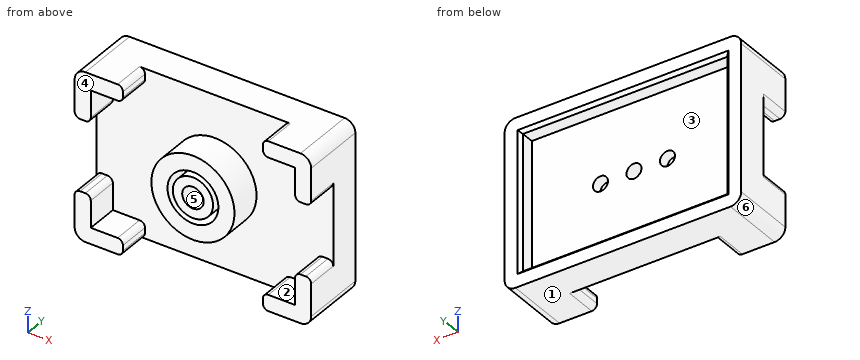
```python
from build123d import *

# Parameters (mm, degrees)
F0_R     = 9.5
F0_R_2   = 7.75
F0_R_3   = 1.4
F0_R_4   = 4.75
F0_R_5   = 3.75
F0_R_6   = 2
F1_DEPTH = 3
F0_W     = 26.1
F0_H     = 3
F0_W_2   = 3
F0_H_2   = 13.3
F2_DEPTH = 6
F3_DEPTH = 1
F4_DEPTH = 6
F5_DEPTH = 6
F6_DEPTH = 6
F7_SIZE  = 0.6
F8_DEPTH = 3
F9_R     = 2
F10_SIZE = 0.4
F11_R    = 1


with BuildPart() as f1:
    # F0 (on Front) → F1 (new body)
    with BuildSketch(Plane.XZ):
        Polygon((-13.05, 12.65), (-19.05, 12.65), (-19.05, 6.65), (-19.05, -6.65), (-19.05, -12.65), (-13.05, -12.65), (13.05, -12.65), (19.05, -12.65), (19.05, -6.65), (19.05, 6.65), (19.05, 12.65), (13.05, 12.65), align=None)
        Circle(F0_R, mode=Mode.SUBTRACT)
        Circle(F0_R)
        Circle(F0_R_2, mode=Mode.SUBTRACT)
        Circle(F0_R_2)
        with Locations((-6.25, 0)):
            Circle(F0_R_3, mode=Mode.SUBTRACT)
        Circle(F0_R_4, mode=Mode.SUBTRACT)
        with Locations((6.25, 0)):
            Circle(F0_R_3, mode=Mode.SUBTRACT)
        Circle(F0_R_4)
        Circle(F0_R_5, mode=Mode.SUBTRACT)
        Circle(F0_R_5)
        Circle(F0_R_6, mode=Mode.SUBTRACT)
    extrude(amount=-F1_DEPTH)

    # F0 (on Front) → F2 (join)
    with BuildSketch(Plane.XZ):
        Polygon((-19.05, 6.65), (-19.05, 12.65), (-13.05, 12.65), (-13.05, 15.65), (-22.05, 15.65), (-22.05, 6.65), align=None)
        Polygon((13.05, 15.65), (13.05, 12.65), (19.05, 12.65), (19.05, 6.65), (22.05, 6.65), (22.05, 15.65), align=None)
        with Locations((0, -14.15)):
            Rectangle(F0_W, F0_H)
        with Locations((0, 14.15)):
            Rectangle(F0_W, F0_H)
        with Locations((-20.55, 0)):
            Rectangle(F0_W_2, F0_H_2)
        Polygon((-19.05, -12.65), (-19.05, -6.65), (-22.05, -6.65), (-22.05, -15.65), (-13.05, -15.65), (-13.05, -12.65), align=None)
        Polygon((22.05, -6.65), (19.05, -6.65), (19.05, -12.65), (13.05, -12.65), (13.05, -15.65), (22.05, -15.65), align=None)
        with Locations((20.55, 0)):
            Rectangle(F0_W_2, F0_H_2)
    extrude(amount=-F2_DEPTH)

    # F0 (on Front) → F3 (join)
    with BuildSketch(Plane.XZ):
        with Locations((-6.25, 0)):
            Circle(F0_R_3)
        with Locations((6.25, 0)):
            Circle(F0_R_3)
    extrude(amount=-F3_DEPTH)

    # F0 (on Front) → F4 (join)
    with BuildSketch(Plane.XZ):
        Circle(F0_R_5)
        Circle(F0_R_6, mode=Mode.SUBTRACT)
    extrude(amount=F4_DEPTH)

    # F0 (on Front) → F5 (join)
    with BuildSketch(Plane.XZ):
        Polygon((-19.05, 6.65), (-19.05, 12.65), (-13.05, 12.65), (-13.05, 15.65), (-22.05, 15.65), (-22.05, 6.65), align=None)
        Polygon((13.05, 15.65), (13.05, 12.65), (19.05, 12.65), (19.05, 6.65), (22.05, 6.65), (22.05, 15.65), align=None)
        Polygon((-19.05, -12.65), (-19.05, -6.65), (-22.05, -6.65), (-22.05, -15.65), (-13.05, -15.65), (-13.05, -12.65), align=None)
        Polygon((22.05, -6.65), (19.05, -6.65), (19.05, -12.65), (13.05, -12.65), (13.05, -15.65), (22.05, -15.65), align=None)
    extrude(amount=F5_DEPTH)

    # F0 (on Front) → F6 (join)
    with BuildSketch(Plane.XZ):
        Circle(F0_R_2)
        with Locations((-6.25, 0)):
            Circle(F0_R_3, mode=Mode.SUBTRACT)
        Circle(F0_R_4, mode=Mode.SUBTRACT)
        with Locations((6.25, 0)):
            Circle(F0_R_3, mode=Mode.SUBTRACT)
        with Locations((-6.25, 0)):
            Circle(F0_R_3)
        with Locations((6.25, 0)):
            Circle(F0_R_3)
    extrude(amount=F6_DEPTH)

    # F7
    f7_edges = [f1.edges().sort_by_distance(p)[0] for p in [
        (0, 6, 12.65),
        (-19.05, 6, 0),
        (19.05, 6, 0),
        (0, 6, -12.65),
    ]]
    chamfer(f7_edges, length=F7_SIZE)

    # F0 (on Front) → F8 (join)
    with BuildSketch(Plane.XZ):
        Circle(F0_R_6)
        Circle(F0_R_3, mode=Mode.SUBTRACT)
    extrude(amount=-F8_DEPTH)

    # F9
    f9_edges = [f1.edges().sort_by_distance(p)[0] for p in [
        (22.05, 0, 15.65),
        (-22.05, 0, 15.65),
        (-22.05, 0, -15.65),
        (22.05, 0, -15.65),
    ]]
    fillet(f9_edges, radius=F9_R)

    # F10
    f10_edges = [f1.edges().sort_by_distance(p)[0] for p in [
        (-1.4, 0, 0),
    ]]
    chamfer(f10_edges, length=F10_SIZE)

    # F11
    f11_edges = [f1.edges().sort_by_distance(p)[0] for p in [
        (-22.05, -3, 6.65),
        (-19.05, -3, 6.65),
        (-13.05, -3, 12.65),
        (-13.05, -3, 15.65),
        (13.05, -3, 12.65),
        (19.05, -3, 6.65),
        (22.05, -3, 6.65),
        (-13.05, -3, -15.65),
        (13.05, -3, -15.65),
        (-22.05, -3, -6.65),
        (-19.05, -3, -6.65),
        (13.05, -3, 15.65),
        (22.05, -3, -6.65),
        (19.05, -3, -6.65),
        (13.05, -3, -12.65),
        (-13.05, -3, -12.65),
    ]]
    fillet(f11_edges, radius=F11_R)


solid = f1.part
```
Input: part model. Units: mm. Frame: model coordinates. Face numbers are marked on the shaded views. A direction names the side the tool comes from. Coordinates: 2 decimals unless noted, no trailing zeros. Write each loop counter-clockwise with the first axis right and the second up, starting at its lowest first coordinate (ties: lowest second). Pieces come first, ordered by that corner, then holes.
1) Mould query, pull axis X, two halves, no side actions, for the marked faces 4, 5 and 6. Classes: pulls with the +X half, pulls with the -X half, needs draft (parallel to the pull), parting line crosses it, or undercut.
2) Pin query (flat end, axial travel): pin 1 Ø0.5 at (y, z) = (-4.5, 14) entering from -X; pin 2 Ø2.5 at (x, z) = (0, 0) entering from +Y; pin 3 Ø3.5 at (x, z) = (6.25, 0) entering from +Y; pin 4 Ø1.4 at (x, z) = (6.5, -0.5) entering from +Y. Return the tip coordinate at first contact, or that it passes through.
3) Section D-D on z = 5.5. Output: boundary loops of the cut face in (x, y), and give its area (3 significant figures).
4) Set-up query: the marked faces 1, 2 and 3. Return all of +Z, -Z, +X, -X, +Y, -Y with unobstructed straight access to the full face (end or side cutting, diameter ignored); none if empty.
5) Material intervals for line 1 along Z through (x, y) = (0, -3.45); line 2 along Z through (x, y) = (6.25, 2.2); line 3 along Z through (x, y) = (16.5, -1.75), sorted ascending.
6) Section B-B on x = 15.5. Output: boundary loops of the cut face in (y, z).
7) Section C-C on y = 2. Output: boundary loops of the cut face in (x, z), and give its area (3 significant figures).
Check result:
1. face 4: needs draft
1. face 5: undercut
1. face 6: pulls with the -X half
2. pin 1: stops at x = -22.05
2. pin 2: passes through
2. pin 3: stops at y = 3
2. pin 4: stops at y = 1
3. outline: (-22.05, 0) - (-5.46, 0) - (-5.46, -6) - (5.46, -6) - (5.46, 0) - (22.05, 0) - (22.05, 6) - (19.65, 6) - (19.05, 5.4) - (19.05, 3) - (-19.05, 3) - (-19.05, 5.4) - (-19.65, 6) - (-22.05, 6) - close
3. area: 215 mm2
4. face 1: -Z, +X, -X, +Y, -Y
4. face 2: -Y
4. face 3: +Y
5. line 1: z = -7.75 to -4.75, -3.75 to -2, 2 to 3.75, 4.75 to 7.75
5. line 2: z = -15.65 to -1.4, 1.4 to 15.65
5. line 3: z = -15.65 to -12.65, 12.65 to 15.65
6. outline: (-6, -15.65) - (6, -15.65) - (6, -13.25) - (5.4, -12.65) - (3, -12.65) - (3, 12.65) - (5.4, 12.65) - (6, 13.25) - (6, 15.65) - (-6, 15.65) - (-6, 12.65) - (0, 12.65) - (0, -12.65) - (-6, -12.65) - close
7. outline: (-22.05, -13.65) arc R2 ccw to (-20.05, -15.65) - (20.05, -15.65) arc R2 ccw to (22.05, -13.65) - (22.05, 13.65) arc R2 ccw to (20.05, 15.65) - (-20.05, 15.65) arc R2 ccw to (-22.05, 13.65) - close; hole circle Ø2.8 at (-6.25, 0); hole circle Ø2.8 at (0, 0); hole circle Ø2.8 at (6.25, 0)
7. area: 1,360 mm2
